Check sheet for the modelled part. Datum: model origin and axes. Units: mm. A direction names the side the tool comes from. Coordinates: 2 decimals unless noted, no trailing zeros. Loops run counter-clockwise (first coordinate to the right, second up) from the corner with the lowest first, then second, coordinate; pieces in that order, holes last. Notation, with made-up numbers: (60.5, 79) - (113.5, 79) arc R22 cw to (113.5, 102) - close; hole circle Ø2 at (0, 83). An arc over 180 degrees is marked (long way). Answer as a JSON object with one key per item and string values. Group by question number.
from build123d import *

# Parameters (mm, degrees)
EXTRUDE_1_DEPTH     = 5
SKETCH_2_R          = 10
EXTRUDE_2_DEPTH     = 15
SKETCH_3_R          = 4
EXTRUDE_3_DEPTH     = 6
SKETCH_4_R          = 5
SKETCH_4_R_2        = 4
EXTRUDE_4_DEPTH     = 1
CHAMFER_1_SIZE      = 0.5
SKETCH_6_R          = 1.3
CUT_EXTRUDE_2_DEPTH = 6
SKETCH_11_R         = 2.2
CUT_EXTRUDE_7_DEPTH = 10
CUT_EXTRUDE_START   = -5
CUT_EXTRUDE_8_DEPTH = 5
CUT_EXTRUDE_START_2 = -3
SKETCH_14_R         = 11.075
SKETCH_14_R_2       = 5
CUT_EXTRUDE_9_DEPTH = 3
EXTRUDE_START       = -1
EXTRUDE_5_DEPTH     = 1
FILLET_1_R          = 2
SKETCH_16_W         = 4.663078912
SKETCH_16_H         = 1.2
EXTRUDE_6_DEPTH     = 4
EXTRUDE_7_DEPTH     = 1
EXTRUDE_8_DEPTH     = 3


with BuildPart() as part:
    # 草图1 → 凸台-拉伸1 (new body)
    with BuildSketch(Plane.XY):
        with BuildLine():
            Line((57.614035088, 6.973016629), (1.052631579, 11.953742793))
            ThreePointArc((1.052631579, 11.953742793), (-12, 0), (1.052631579, -11.953742793))
            Line((1.052631579, -11.953742793), (57.614035088, -6.973016629))
            ThreePointArc((57.614035088, -6.973016629), (64, 0), (57.614035088, 6.973016629))
        make_face()
    extrude(amount=EXTRUDE_1_DEPTH)

    # 草图2 → 凸台-拉伸2 (add)
    with BuildSketch(Plane.XY.offset(5)):
        Circle(SKETCH_2_R)
    extrude(amount=EXTRUDE_2_DEPTH)

    # 草图3 → 凸台-拉伸3 (add)
    with BuildSketch(Plane(origin=(0, 0, 0), x_dir=(-1, 0, 0), z_dir=(0, 0, -1))):
        with Locations((-57, 0)):
            Circle(SKETCH_3_R)
    extrude(amount=EXTRUDE_3_DEPTH)

    # 草图4 → 凸台-拉伸4 (add)
    with BuildSketch(Plane(origin=(0, 0, 0), x_dir=(-1, 0, 0), z_dir=(0, 0, -1))):
        with Locations(Location((-57, 0, 0), (0, 0, 180))):
            Circle(SKETCH_4_R)
        with Locations((-57, 0)):
            Circle(SKETCH_4_R_2, mode=Mode.SUBTRACT)
    extrude(amount=EXTRUDE_4_DEPTH)

    # 倒角1
    chamfer_1_edges = [part.edges().sort_by_distance(p)[0] for p in [
        (-10, 0, 20),
        (61, 0, -6),
        (52, 0, -1),
    ]]
    chamfer(chamfer_1_edges, length=CHAMFER_1_SIZE)

    # 草图6 → 切除-拉伸2 (cut)
    with BuildSketch(Plane.XY.offset(20)):
        with Locations((0, 7)):
            Circle(SKETCH_6_R)
        with Locations((7, 0)):
            Circle(SKETCH_6_R)
        with Locations((0, -7)):
            Circle(SKETCH_6_R)
        with Locations((-7, 0)):
            Circle(SKETCH_6_R)
    extrude(amount=-CUT_EXTRUDE_2_DEPTH, mode=Mode.SUBTRACT)

    # 草图11 → 切除-拉伸7 (cut)
    with BuildSketch(Plane(origin=(0, 0, -6), x_dir=(-1, 0, 0), z_dir=(0, 0, -1))):
        with Locations((-57, 0)):
            Circle(SKETCH_11_R)
    extrude(amount=-CUT_EXTRUDE_7_DEPTH, mode=Mode.SUBTRACT)

    # 草图12 → 切除-拉伸8 (cut)
    with BuildSketch(Plane.XY.offset(5).offset(CUT_EXTRUDE_START)):
        with BuildLine():
            Line((57.438596491, 4.980726164), (7.48487293, 9.379588329))
            ThreePointArc((7.48487293, 9.379588329), (10.812457518, 5.204878713), (12, 0))
            ThreePointArc((12, 0), (10.812457518, -5.204878713), (7.48487293, -9.379588329))
            Line((7.48487293, -9.379588329), (57.438596491, -4.980726164))
            ThreePointArc((57.438596491, -4.980726164), (52, 0), (57.438596491, 4.980726164))
        make_face()
    extrude(amount=CUT_EXTRUDE_8_DEPTH, mode=Mode.SUBTRACT)

    # 草图14 → 切除-拉伸9 (cut)
    with BuildSketch(Plane(origin=(0, 0, 0), x_dir=(-1, 0, 0), z_dir=(0, 0, -1)).offset(CUT_EXTRUDE_START_2)):
        with Locations((-57, 0)):
            Circle(SKETCH_14_R)
        with Locations(Location((-57, 0, 0), (0, 0, 95.032413496))):
            Circle(SKETCH_14_R_2, mode=Mode.SUBTRACT)
    extrude(amount=CUT_EXTRUDE_9_DEPTH, mode=Mode.SUBTRACT)

    # 草图15 → 凸台-拉伸5 (add)
    with BuildSketch(Plane.XY.offset(5).offset(EXTRUDE_START)):
        with BuildLine():
            Line((1.052631579, -11.953742793), (57.614035088, -6.973016629))
            ThreePointArc((57.614035088, -6.973016629), (64, 0), (57.614035088, 6.973016629))
            Line((57.614035088, 6.973016629), (1.052631579, 11.953742793))
            ThreePointArc((1.052631579, 11.953742793), (-12, 0), (1.052631579, -11.953742793))
        make_face()
    extrude(amount=EXTRUDE_5_DEPTH)

    # 圆角1
    # the kernel refuses this fillet: 2 mm, written as the material it takes off along each edge
    with BuildSketch(Plane(origin=(49.064832266, -7.725848694, -8.249501326), x_dir=(-0.6163800221199659, 0.7874488353736963, 0), z_dir=(0, 0, 1))) as fillet_1_piece_1:
        with BuildLine():
            CenterArc((3.475122508, 1.676963653), FILLET_1_R, 146.980149767, 90)
            Line((1.798158856, 2.766822775), (0, 0))
            ThreePointArc((0, 0), (1.192631693, 0.064402621), (2.385263386, 0))
        make_face()
    extrude(amount=11.249501326, mode=Mode.SUBTRACT)
    with BuildSketch(Plane(origin=(49.064832266, 7.725848694, -8.249501326), x_dir=(-0.9961452327423431, 0.08771929824561424, 0), z_dir=(0, 0, 1))) as fillet_1_piece_2:
        with BuildLine():
            CenterArc((3.29980053, 2), FILLET_1_R, 180, 90)
            ThreePointArc((1.29980053, 2), (0.703900692, 0.964905108), (0, 0))
            Line((0, 0), (3.29980053, 0))
        make_face()
    extrude(amount=11.249501326, mode=Mode.SUBTRACT)

    # 草图16 → 切除-旋转1 (revolve, cut)
    with BuildSketch(Plane(origin=(0, 0, 0), x_dir=(1, 0, 0), z_dir=(0, 1, 0))):
        with Locations((11.581539456, -17.6)):
            Rectangle(SKETCH_16_W, SKETCH_16_H)
    revolve(axis=Axis((0, 0, 20), (0, 0, -1)), mode=Mode.SUBTRACT)

    # 草图17 → 凸台-拉伸6 (add)
    # profile 1 of 2: a face of its own
    with BuildSketch(Plane(origin=(0, 0, 4), x_dir=(-1, 0, 0), z_dir=(0, 0, -1))):
        with BuildLine():
            ThreePointArc((-7.48487293, -9.379588329), (-12, 0), (-7.48487293, 9.379588329))
            Line((-7.48487293, 9.379588329), (-47.594603568, 5.847575819))
            ThreePointArc((-47.594603568, 5.847575819), (-45.925, 0), (-47.594603568, -5.847575819))
            Line((-47.594603568, -5.847575819), (-7.48487293, -9.379588329))
        make_face()
        with BuildLine():
            Line((-43.563456974, -2.155807668), (-43.563456974, 2.155807668))
            Line((-43.563456974, 2.155807668), (-15.344753505, 4.640711258))
            ThreePointArc((-15.344753505, 4.640711258), (-16.031146594, 0), (-15.344753505, -4.640711258))
            Line((-15.344753505, -4.640711258), (-43.563456974, -2.155807668))
        make_face(mode=Mode.SUBTRACT)
    # profile 2 of 2: a face of its own
    with BuildSketch(Plane(origin=(0, 0, 4), x_dir=(-1, 0, 0), z_dir=(0, 0, -1))):
        with BuildLine():
            ThreePointArc((-15.344753505, 4.640711258), (-16.031146594, 0), (-15.344753505, -4.640711258))
            Line((-15.344753505, -4.640711258), (-43.563456974, -2.155807668))
            Line((-43.563456974, -2.155807668), (-43.563456974, 2.155807668))
            Line((-43.563456974, 2.155807668), (-15.344753505, 4.640711258))
        make_face()
    extrude(amount=EXTRUDE_6_DEPTH)

    # 草图18 → 凸台-拉伸7 (add)
    with BuildSketch(Plane(origin=(0, 0, 4), x_dir=(-1, 0, 0), z_dir=(0, 0, -1))):
        with BuildLine():
            Line((-47.594603568, 5.847575819), (-57.438596491, 4.980726164))
            ThreePointArc((-57.438596491, 4.980726164), (-52, 0), (-57.438596491, -4.980726164))
            Line((-57.438596491, -4.980726164), (-47.594603568, -5.847575819))
            ThreePointArc((-47.594603568, -5.847575819), (-45.925, 0), (-47.594603568, 5.847575819))
        make_face()
    extrude(amount=EXTRUDE_7_DEPTH)

    # 草图19 → 凸台-拉伸8 (add)
    with BuildSketch(Plane.XY.offset(5)):
        with BuildLine():
            Line((28.442097172, -9.541860848), (57.614035088, -6.973016629))
            ThreePointArc((57.614035088, -6.973016629), (64, 0), (57.614035088, 6.973016629))
            Line((57.614035088, 6.973016629), (28.442097172, 9.541860848))
            ThreePointArc((28.442097172, 9.541860848), (30, 0), (28.442097172, -9.541860848))
        make_face()
    extrude(amount=EXTRUDE_8_DEPTH)


solid = part.part
1. Sectioned sample at C-C on z = 8.75. Record the cut outline in (x, y), plus the area to 3 significant figures.
2. Release check for a two-part mould opening along Y. For faces 1 (the face through (8.24, 0.39, 17.04)), 2 (the face through (46, 0, 8)), 3 (the face through (-2.17, -9.76, 10.92)) record: released by +Y, released by -Y, zero draft, split by the parting line, or undercut.
3. Material ranges on line 1 (Y direction, x = 0, z = 15.35); line 2 (Y direction, x = 0, z = 18.1); line 3 (Y direction, x = 57, z = 0.5), recorded low to high.
4. Access from +Z, -Z, +X, -X, +Y, -Y to the whole of each face (thin tool, end or side, straight path). Record for faces 4 (the face through (-3, 9, 17)), 5 (the face through (64, 0, 5)), 6 (the face through (-0.28, -8.27, 17.04)), 7 (the face through (54, 3, -1)).
5. Gauge pin test, flat ends, axial feed: pin 1 (2 mm diameter, centred on x = 26, y = -1.5, fed in from -Z); pin 2 (2 mm diameter, centred on x = 56.5, y = -0.5, fed in from -Z); pin 3 (8 mm diameter, centred on x = 53.5, z = 5, fed in from -Y). Record the tip position at first contact, or that the pin passes through.
6. Sectioned sample at D-D on x = 23. Record the cut outline in (y, z).
7. Sectioned sample at B-B on z = -3.5. Record the cut outline in (x, y), plus the area to 3 significant figures.
8. Sectioned sample at A-A on x = 0. Record the cut outline in (y, z), plus the area to 3 significant figures.
Answers follow:
{
 "1": {"outline": "circle Ø20 at (0, 0)", "area": "314 mm^2"},
 "2": {"face 1": "undercut", "face 2": "zero draft", "face 3": "split by the parting line"},
 "3": {"line 1": "y = -10 to -8.3, -5.7 to 5.7, 8.3 to 10", "line 2": "y = -9.25 to -8.3, -5.7 to 5.7, 8.3 to 9.25", "line 3": "y = -5 to -2.2, 2.2 to 5"},
 "4": {"face 4": "none", "face 5": "+Z, -Z, +X", "face 6": "+Z", "face 7": "-Z"},
 "5": {"pin 1": "stops at z = 0", "pin 2": "stops at z = 4", "pin 3": "stops at y = -7.69"},
 "6": {"outline": "(-10.02, 0) - (10.02, 0) - (10.02, 5) - (-10.02, 5) - close"},
 "7": {"outline": "circle Ø8 at (57, 0); hole circle Ø4.4 at (57, 0)", "area": "35.1 mm^2"},
 "8": {"outline": "(-12, 0) - (12, 0) - (12, 5) - (10, 5) - (10, 17) - (9.25, 17) - (9.25, 18.2) - (10, 18.2) - (10, 19.5) - (9.5, 20) - (8.3, 20) - (8.3, 14) - (5.7, 14) - (5.7, 20) - (-5.7, 20) - (-5.7, 14) - (-8.3, 14) - (-8.3, 20) - (-9.5, 20) - (-10, 19.5) - (-10, 18.2) - (-9.25, 18.2) - (-9.25, 17) - (-10, 17) - (-10, 5) - (-12, 5) - close", "area": "387 mm^2"}
}
